Geometry: final body of the model. Coordinates: model frame, mm. Face numbers are marked on the shaded views. A direction names the side the tool comes from. Give positions to 0.01 mm unless a question says otherwise; leave off trailing zeros. Order: outer loops, then holes, each group sorted by start corner. A loop starts at its lowest first (then second) coordinate and runs counter-clockwise, first axis right, second up. Notation, with made-up numbers: M -7.5,63 L 7.5,63 A17 cw 7.5,91 Z; hole C 81,69 d5. An arc over 180 degrees is marked long. One line per item, written item: value. Start each with the question number.
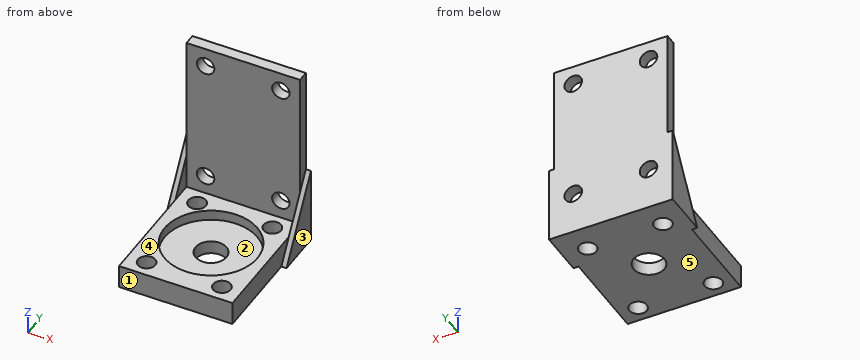
```python
from build123d import *

# Parameters (mm, degrees)
SKETCH1_W           = 22
SKETCH1_H           = 27
BOSS_EXTRUDE1_DEPTH = 4.577
SKETCH2_W           = 22
SKETCH2_H           = 2.167
BOSS_EXTRUDE2_DEPTH = 31.43
SKETCH5_R           = 1.7
CUT_EXTRUDE1_DEPTH  = 49.961024683
SKETCH6_R           = 1.7
CUT_EXTRUDE2_DEPTH  = 49.961024683
SKETCH7_R           = 1.7
CUT_EXTRUDE3_DEPTH  = 49.961024683
SKETCH8_R           = 1.7
CUT_EXTRUDE4_DEPTH  = 49.961024683
BOSS_EXTRUDE6_DEPTH = 1
BOSS_EXTRUDE7_DEPTH = 1
SKETCH10_R          = 1.7
CUT_EXTRUDE6_DEPTH  = 48.390346063
SKETCH10_7_R        = 1.7
CUT_EXTRUDE7_DEPTH  = 10
SKETCH10_8_R        = 1.7
CUT_EXTRUDE8_DEPTH  = 10
SKETCH10_9_R        = 1.7
CUT_EXTRUDE9_DEPTH  = 10
SKETCH10_10_R       = 9
CUT_EXTRUDE10_DEPTH = 2
SKETCH10_12_R       = 3
CUT_EXTRUDE11_DEPTH = 48.390346063


with BuildPart() as part:
    # Sketch1 → Boss-Extrude1 (new body)
    with BuildSketch(Plane.XY):
        with Locations((11, 13.5)):
            Rectangle(SKETCH1_W, SKETCH1_H)
    extrude(amount=BOSS_EXTRUDE1_DEPTH)

    # Sketch2 → Boss-Extrude2 (add)
    with BuildSketch(Plane.XY.offset(4.577)):
        with Locations((11, 25.9165)):
            Rectangle(SKETCH2_W, SKETCH2_H)
    extrude(amount=BOSS_EXTRUDE2_DEPTH)

    # Sketch5 → Cut-Extrude1 (cut, through all)
    with BuildSketch(Plane.XZ.offset(-24.833)):
        with Locations(Location((3.7, 8.277, 0), (0, 0, 270))):
            Circle(SKETCH5_R)
    extrude(amount=-CUT_EXTRUDE1_DEPTH, mode=Mode.SUBTRACT)

    # Sketch6 → Cut-Extrude2 (cut, through all)
    with BuildSketch(Plane.XZ.offset(-24.833)):
        with Locations(Location((18.3, 8.277, 0), (0, 0, 270))):
            Circle(SKETCH6_R)
    extrude(amount=-CUT_EXTRUDE2_DEPTH, mode=Mode.SUBTRACT)

    # Sketch7 → Cut-Extrude3 (cut, through all)
    with BuildSketch(Plane.XZ.offset(-24.833)):
        with Locations(Location((3.7, 32.307, 0), (0, 0, 270))):
            Circle(SKETCH7_R)
    extrude(amount=-CUT_EXTRUDE3_DEPTH, mode=Mode.SUBTRACT)

    # Sketch8 → Cut-Extrude4 (cut, through all)
    with BuildSketch(Plane.XZ.offset(-24.833)):
        with Locations(Location((18.3, 32.307, 0), (0, 0, 270))):
            Circle(SKETCH8_R)
    extrude(amount=-CUT_EXTRUDE4_DEPTH, mode=Mode.SUBTRACT)

    # Sketch12 → Boss-Extrude6 (add)
    with BuildSketch(Plane(origin=(22, 0, 0), x_dir=(0, 0, -1), z_dir=(1, 0, 0))):
        Polygon((0, 27), (-15, 27), (0, 18), align=None)
    extrude(amount=BOSS_EXTRUDE6_DEPTH)

    # Sketch13 → Boss-Extrude7 (add)
    with BuildSketch(Plane.ZY):
        Polygon((0, 27), (0, 18), (15, 27), align=None)
    extrude(amount=BOSS_EXTRUDE7_DEPTH)

    # Sketch10 → Cut-Extrude6 (cut, through all)
    with BuildSketch(Plane.XY.offset(4.577)):
        with Locations((18.3, 21.7)):
            Circle(SKETCH10_R)
    extrude(amount=-CUT_EXTRUDE6_DEPTH, mode=Mode.SUBTRACT)

    # Sketch10_7 → Cut-Extrude7 (cut)
    with BuildSketch(Plane.XY.offset(4.577)):
        with Locations((3.7, 21.7)):
            Circle(SKETCH10_7_R)
    extrude(amount=-CUT_EXTRUDE7_DEPTH, mode=Mode.SUBTRACT)

    # Sketch10_8 → Cut-Extrude8 (cut)
    with BuildSketch(Plane.XY.offset(4.577)):
        with Locations((18.3, 3.133)):
            Circle(SKETCH10_8_R)
    extrude(amount=-CUT_EXTRUDE8_DEPTH, mode=Mode.SUBTRACT)

    # Sketch10_9 → Cut-Extrude9 (cut)
    with BuildSketch(Plane.XY.offset(4.577)):
        with Locations((3.7, 3.133)):
            Circle(SKETCH10_9_R)
    extrude(amount=-CUT_EXTRUDE9_DEPTH, mode=Mode.SUBTRACT)

    # Sketch10_10 → Cut-Extrude10 (cut)
    with BuildSketch(Plane.XY.offset(4.577)):
        with Locations((10.991429636, 13)):
            Circle(SKETCH10_10_R)
    extrude(amount=-CUT_EXTRUDE10_DEPTH, mode=Mode.SUBTRACT)

    # Sketch10_12 → Cut-Extrude11 (cut, through all)
    with BuildSketch(Plane.XY.offset(4.577)):
        with Locations((10.991429636, 13)):
            Circle(SKETCH10_12_R)
    extrude(amount=-CUT_EXTRUDE11_DEPTH, mode=Mode.SUBTRACT)


solid = part.part
```
Q1. Contact query for flat-ended pins moving along their axis: pin 1 (1.2 mm diameter, centred on y = 22.5, z = 9.5, fed in from -X); pin 2 (6.5 mm diameter, centred on x = 12, z = 25.5, fed in from -Y); pin 3 (2.5 mm diameter, centred on y = 12, z = 2.5, fed in from -X); pin 4 (4.5 mm diameter, centred on x = 18.3, y = 3.133, fed in from +Z). Output: stop coordinate, or through.
Q2. Section query A-A on y = 13. Return loops of the section in (x, z), and give its area (3 significant figures).
Q3. Section query B-B on x = 3.7. Return loops of the section in (y, z), and give its area (3 significant figures).
Q4. Section query D-D on x = 20.5. Return loops of the section in (y, z).
Q5. Section query C-C on z = 14.5. Return loops of the section in (x, y).
Q6. Mould query, pull axis X, two halves, no side actions, for the marked faces 1, 2 and 3. Classes: +X half, -X half, draft (parallel to the pull), parting line (faces both ways), or undercut.
Q7. Ray query, line 1 along Z through (x, y) = (4, 25.75); line 2 along Y through (x, z) = (16.75, 25.5); line 3 along Z through (x, y) = (6.5, 9.75). Return the intervals inside material, ascending. Write a range as [from, to].
Q8. Set-up query: the marked faces 4 and 5. Return all of +Z, -Z, +X, -X, +Y, -Y with unobstructed straight access to the full face (end or side cutting, diameter ignored); none if empty.
Results below:
1. pin 1: through
1. pin 2: y = 24.83
1. pin 3: x = 0
1. pin 4: z = 4.58
2. outline: M 0,0 L 7.99,0 L 7.99,2.58 L 1.99,2.58 L 1.99,4.58 L 0,4.58 Z; M 13.99,0 L 22,0 L 22,4.58 L 19.99,4.58 L 19.99,2.58 L 13.99,2.58 Z
2. area: 49.2 mm2
3. outline: M 0,0 L 1.43,0 L 1.43,4.58 L 0,4.58 Z; M 4.83,0 L 20,0 L 20,4.58 L 18.28,4.58 L 18.28,2.58 L 7.72,2.58 L 7.72,4.58 L 4.83,4.58 Z; M 23.4,0 L 27,0 L 27,6.58 L 24.83,6.58 L 24.83,4.58 L 23.4,4.58 Z; M 24.83,9.98 L 27,9.98 L 27,30.61 L 24.83,30.61 Z; M 24.83,34.01 L 27,34.01 L 27,36.01 L 24.83,36.01 Z
3. area: 125 mm2
4. outline: M 0,0 L 27,0 L 27,36.01 L 24.83,36.01 L 24.83,4.58 L 0,4.58 Z
5. outline: M -1,26.7 L 0,26.7 L 0,24.83 L 22,24.83 L 22,26.7 L 23,26.7 L 23,27 L -1,27 Z
6. face 1: draft
6. face 2: undercut
6. face 3: +X half
7. line 1: [0, 6.6], [9.95, 30.63], [33.98, 36.01]
7. line 2: [24.83, 27]
7. line 3: [0, 2.58]
8. face 4: +Z, -Y
8. face 5: -Z, +X, -X, +Y, -Y
